Here's how the part is built. I have some questions about the finished solid (model axes, mm). Face numbers are marked on the shaded views. A direction names the side the tool comes from. Coordinates: 2 decimals unless noted, no trailing zeros. Loops run counter-clockwise (first coordinate to the right, second up) from the corner with the lowest first, then second, coordinate; pieces in that order, holes last. Notation, with made-up numbers: M -8.75,53.25 L -1.75,53.25 A21 ccw -1.75,60.25 Z; hole C 26,73.5 d6. An arc over 180 degrees is marked long. Use one line per item in the form item = value. Start each with the question number.
(1) Please list where these lines run through material, in increasing order: L1, parallel to Z at x = 839, y = 212 (3 decimals); L2, parallel to X at y = 34, z = -114 (3 decimals); L3, parallel to Y at x = 629, z = -176 (3 decimals).
(2) Imagine slicing it at B-B, the plane y = 284. Please give me the cut outline in (x, z) (3 decimals), and give its area (3 significant figures).
(3) Imagine slicing it at C-C, the plane z = -469. Please give me the cut outline in (x, y) (3 decimals), and give its area (3 significant figures).
(4) Thinking about a two-plate mould opening in X: for the marked faces 3, 4 and 5, which applies, +X half, -X half, draft (parallel to the pull), parting line (faces both ways), or undercut?
(5) On a 3-axis mill with a long thin cutter (end or side, diameter ignored), from which of +Z, -Z, +X, -X, +Y, -Y can I reach the whole of each face in a straight line? I mean the marked faces 1 and 2. Say none if no direction works.
(6) Imagine slicing it at D-D, the plane x = 1219. Please give me the cut outline in (y, z) (3 decimals).
(7) Imagine slicing it at A-A, the plane x = 685. Please give me the cut outline in (y, z) (3 decimals).
(8) Will this pin go through, and if not, where does the flat tip stop? P1, Ø2, axis at x = 178.5, z = -263, coming from the +Y side (3 decimals).
```python
from build123d import *

# Parameters (mm, degrees)
SKETCH1_W           = 1370
SKETCH1_H           = 837.05
BOSS_EXTRUDE1_DEPTH = 350
SHELL1_T            = -9.525
SKETCH3_W           = 287.4
SKETCH3_H           = 82
CUT_EXTRUDE1_DEPTH  = 9.525
CUT_EXTRUDE2_REACH  = 1645.184
SKETCH7_R           = 100


with BuildPart() as part:
    # Sketch1 → Boss-Extrude1 (new body)
    with BuildSketch(Plane(origin=(0, 0, 0), x_dir=(1, 0, 0), z_dir=(0, 1, 0))):
        with Locations((685, 418.525)):
            Rectangle(SKETCH1_W, SKETCH1_H)
    extrude(amount=BOSS_EXTRUDE1_DEPTH)

    # Shell1
    shell1_openings = [part.faces().sort_by_distance(p)[0] for p in [
        (685, 350, -418.525),
    ]]
    offset(amount=SHELL1_T, openings=shell1_openings, kind=Kind.INTERSECTION)

    # Sketch3 → Cut-Extrude1 (cut)
    with BuildSketch(Plane.XY):
        with Locations((158.7, 201.1)):
            Rectangle(SKETCH3_W, SKETCH3_H)
    extrude(amount=-CUT_EXTRUDE1_DEPTH, mode=Mode.SUBTRACT)

    # Sketch7 → Cut-Extrude2 (cut, up to next)
    with BuildSketch(Plane.XZ, mode=Mode.PRIVATE) as cut_extrude2_sk1:
        with Locations(Location((685, -418.525, 0), (0, 0, 270))):
            Circle(SKETCH7_R)
    cut_extrude2_tool1 = extrude(cut_extrude2_sk1.sketch, amount=-CUT_EXTRUDE2_REACH, mode=Mode.PRIVATE) & part.part
    add(cut_extrude2_tool1.solids().sort_by_distance((685, 0, -418.525))[0], mode=Mode.SUBTRACT)


solid = part.part
```
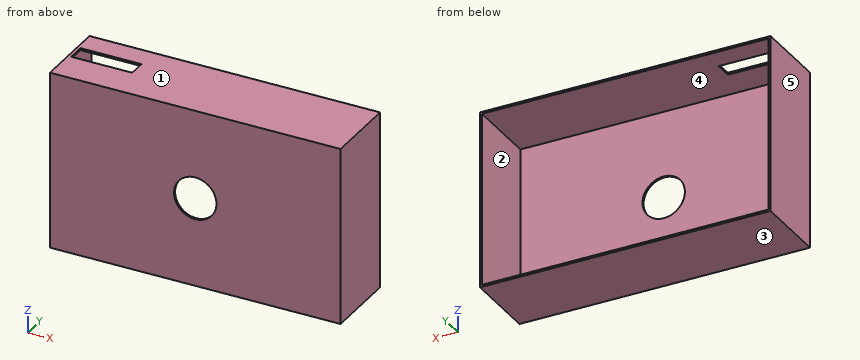
Answer:
q1.L1 = -837.05 to -827.525, -9.525 to 0
q1.L2 = 0 to 9.525, 1360.475 to 1370
q1.L3 = 0 to 9.525
q2.outline = M 0,-837.05 L 1370,-837.05 L 1370,0 L 0,0 Z; hole M 9.525,-827.525 L 1360.475,-827.525 L 1360.475,-9.525 L 9.525,-9.525 Z
q2.area = 41,700 mm²
q3.outline = M 0,0 L 598.673,0 L 598.673,9.525 L 9.525,9.525 L 9.525,350 L 0,350 Z; M 771.327,0 L 1370,0 L 1370,350 L 1360.475,350 L 1360.475,9.525 L 771.327,9.525 Z
q3.area = 17,900 mm²
q4.face_3 = draft
q4.face_4 = undercut
q4.face_5 = -X half
q5.face_1 = +Z, +X, -X, +Y, -Y
q5.face_2 = +Y
q6.outline = M 0,-837.05 L 350,-837.05 L 350,-827.525 L 9.525,-827.525 L 9.525,-9.525 L 350,-9.525 L 350,0 L 0,0 Z
q7.outline = M 0,-837.05 L 350,-837.05 L 350,-827.525 L 9.525,-827.525 L 9.525,-518.525 L 0,-518.525 Z; M 0,-318.525 L 9.525,-318.525 L 9.525,-9.525 L 350,-9.525 L 350,0 L 0,0 Z
q8.P1 = 9.525
